```python
from build123d import *

# Parameters (mm, degrees)
SKETCH1_W           = 25
SKETCH1_H           = 25
SKETCH1_R           = 2.2225
BOSS_EXTRUDE1_DEPTH = 10
SKETCH2_R           = 3.937
CUT_EXTRUDE3_DEPTH  = 4.318
BOSS_EXTRUDE2_DEPTH = 12
FILLET1_R           = 3
CUT_EXTRUDE4_REACH  = 38.454
SKETCH3_R           = 1.7
FILLET2_R           = 3


with BuildPart() as part:
    # Sketch1 → Boss-Extrude1 (new body)
    with BuildSketch(Plane.XY):
        Rectangle(SKETCH1_W, SKETCH1_H)
        with Locations((-5.563, 5.0876)):
            Circle(SKETCH1_R, mode=Mode.SUBTRACT)
        with Locations((7.137, -6.0376)):
            Circle(SKETCH1_R, mode=Mode.SUBTRACT)
    extrude(amount=BOSS_EXTRUDE1_DEPTH)

    # Sketch2 → Cut-Extrude3 (cut)
    with BuildSketch(Plane.XY.offset(10)):
        with Locations((-5.563, 5.0876)):
            Circle(SKETCH2_R)
        with Locations((7.137, -6.0376)):
            Circle(SKETCH2_R)
    extrude(amount=-CUT_EXTRUDE3_DEPTH, mode=Mode.SUBTRACT)

    # 3DSketch1 → Boss-Extrude2 (add, along a direction that is not the sketch's normal)
    with BuildSketch(Plane(origin=(-12.5, -12.5, 0), x_dir=(0, 0.5144957554275265, 0.8574929257125442), z_dir=(-0.999897134802458, -0.012298966175927167, 0.007379379705556298))):
        Polygon((0, 0), (3.086974533, 5.144957554), (11.66190379, 0), (8.574929257, -5.144957554), align=None)
    boss_extrude2 = extrude(amount=BOSS_EXTRUDE2_DEPTH, dir=(-1, 0, 0))

    # Mirror1: Boss-Extrude2 across plane
    add(boss_extrude2.mirror(Plane(origin=(0, 0, 0), x_dir=(0, 0, 1), z_dir=(1, 0, 0))))

    # Fillet1
    fillet1_edges = [part.edges().sort_by_distance(p)[0] for p in [
        (12.5, 12.5, 5),
        (-12.5, 12.5, 5),
    ]]
    fillet(fillet1_edges, radius=FILLET1_R)

    # Cut-Extrude4: up to this plane
    cut_extrude4_end = Plane(origin=(-12.573793797, -6.500453817, 0.00027229), z_dir=(0, 0.9999999989701944, -4.538294048436099e-05))
    # Sketch3 → Cut-Extrude4 (cut, up to the surface)
    with BuildSketch(Plane.XZ.offset(12.5), mode=Mode.PRIVATE) as cut_extrude4_sk1:
        with Locations(Location((-18.462939729, 4.999863855, 0), (0, 0, 270))):
            Circle(SKETCH3_R)
    cut_extrude4_tool1 = split(extrude(cut_extrude4_sk1.sketch, amount=-CUT_EXTRUDE4_REACH, mode=Mode.PRIVATE), bisect_by=cut_extrude4_end, keep=Keep.BOTH, mode=Mode.PRIVATE)
    add(cut_extrude4_tool1.solids().sort_by_distance((-18.46294, -12.5, 4.999864))[0], mode=Mode.SUBTRACT)
    # Sketch3 → Cut-Extrude4 (cut, up to the surface)
    with BuildSketch(Plane.XZ.offset(12.5), mode=Mode.PRIVATE) as cut_extrude4_sk2:
        with Locations(Location((18.462939729, 4.999863855, 0), (0, 0, 270))):
            Circle(SKETCH3_R)
    cut_extrude4_tool2 = split(extrude(cut_extrude4_sk2.sketch, amount=-CUT_EXTRUDE4_REACH, mode=Mode.PRIVATE), bisect_by=cut_extrude4_end, keep=Keep.BOTH, mode=Mode.PRIVATE)
    add(cut_extrude4_tool2.solids().sort_by_distance((18.46294, -12.5, 4.999864))[0], mode=Mode.SUBTRACT)

    # Fillet2
    fillet2_edges = [part.edges().sort_by_distance(p)[0] for p in [
        (-24.536896899, -6.500226909, 5.000136145),
        (24.536896899, -6.500226909, 5.000136145),
    ]]
    fillet(fillet2_edges, radius=FILLET2_R)


solid = part.part
```
Design review of the part built by this model. Coordinates are the model's own, in mm. A direction names the side the tool comes from. Give positions to 0.01 mm unless a question says otherwise; leave off trailing zeros. Write each loop counter-clockwise with the first axis right and the second up, starting at its lowest first coordinate (ties: lowest second). Pieces come first, ordered by that corner, then holes.
(1) Mouldability with a two-part tool opening along Y and no side actions: class faces 3 (the face through (20.15, -9.54, 5.22)), 4 (the face through (10.77, -7.55, 7.87)), 5 (the face through (0, -12.5, 5)) as +Y half, -Y half, draft (parallel to the pull), parting line (faces both ways), or undercut.
Checked values:
face 3: draft
face 4: undercut
face 5: -Y half
(2) Add section D-D (y = 2.25). Give the boundary of the cut face in (x, z).
Checked values:
outline: (-12.5, 0) - (12.5, 0) - (12.5, 10) - (-2.83, 10) - (-2.83, 5.68) - (-8.29, 5.68) - (-8.29, 10) - (-12.5, 10) - close
(3) Tool access review of faces 1 (the face through (-6.416, 1.244, 7.871)), 2 (the face through (6.66, -8.21, 2.8)): name each direction out of +Z, -Z, +X, -X, +Y, -Y from which nothing blocks a thin tool from reaching the whole face with its end or side.
Checked values:
face 1: +Z
face 2: +Z, -Z
(4) Add section C-C (z = 4.75). Give the number of separate pieces and of enclosed holes in the cut face, and give its area (3 significant figures).
Checked values:
separate pieces: 3
enclosed holes: 2
area: 690 mm2
(5) Clearance check with flat-ended pins moving along their axes: pin 1 Ø4 at (y, z) = (-8, 3.5) entering from +X; pin 2 Ø1.5 at (y, z) = (-5, 5) entering from -X; pin 3 Ø4 at (x, y) = (-5.5, 4.5) entering from +Z. State where each tip first meets the part, or that it passes through.
Checked values:
pin 1: stops at x = 24.52
pin 2: stops at x = -12.5
pin 3: stops at z = 5.68
(6) Wall thickness on line 1 along X through (y, z) = (5.25, 4.5); line 2 along X through (y, z) = (-10.5, 6); line 3 along Y through (x, z) = (-19.5, 3.5): over which ranges is each line inside the solid? List them lowest first.
Checked values:
line 1: x = -12.5 to -7.78, -3.35 to 12.5
line 2: x = -24.48 to -19.84, -17.09 to 17.09, 19.84 to 24.48
line 3: y = -12.5 to -6.5
(7) Add section B-B (y = 6). Give the boundary of the cut face in (x, z).
Checked values:
outline: (-12.5, 0) - (-7.59, 0) - (-7.59, 5.68) - (-9.39, 5.68) - (-9.39, 10) - (-12.5, 10) - close; (-3.54, 0) - (12.5, 0) - (12.5, 10) - (-1.73, 10) - (-1.73, 5.68) - (-3.54, 5.68) - close
(8) Add section A-A (x = -6). Give the boundary of the cut face in (y, z).
Checked values:
outline: (-12.5, 0) - (2.91, 0) - (2.91, 5.68) - (1.17, 5.68) - (1.17, 10) - (-12.5, 10) - close; (7.27, 0) - (12.5, 0) - (12.5, 10) - (9, 10) - (9, 5.68) - (7.27, 5.68) - close
